from build123d import *

# Parameters (mm, degrees)
F0_W     = 9
F0_H     = 5.1
F1_DEPTH = 0.5
F2_SIZE  = 0.5
F3_SIZE  = 0.1


with BuildPart() as f1:
    # F0 (on Front) → F1 (new body, symmetric)
    with BuildSketch(Plane.XZ):
        with Locations((4.5, 2.55)):
            Rectangle(F0_W, F0_H)
    extrude(amount=F1_DEPTH, both=True)

    # F2
    f2_edges = [f1.edges().sort_by_distance(p)[0] for p in [
        (4.5, 0.5, 0),
    ]]
    chamfer(f2_edges, length=F2_SIZE)

    # F3
    f3_edges = [f1.edges().sort_by_distance(p)[0] for p in [
        (4.5, -0.5, 0),
    ]]
    chamfer(f3_edges, length=F3_SIZE)


solid = f1.part
Design review of the part built by this model. Coordinates are the model's own, in mm. Give positions to 0.01 mm unless a question says otherwise; leave off trailing zeros. Loops run counter-clockwise (first coordinate to the right, second up) from the corner with the lowest first, then second, coordinate; pieces in that order, holes last. Notation, with made-up numbers: M 69,64.25 L 91,64.25 A17 ccw 91,71.25 Z; hole C -23.5,7 d5. An arc over 180 degrees is marked long. One line per question, with ' | ' between items. Start each with the question number.
1. To check wall thickness, follow L1, parallel to Y at x = 8.75, z = 0.4; L2, parallel to Z at x = 1.5, y = 0.05; L3, parallel to Z at x = 6.5, y = 0.35. State the ranges of each line that lie inside material, in increasing order.
2. The part is to be moulded in two halves that separate along Z. For faces 1 (the face through (4, 0, 5.1)), 2 (the face through (4, -0.5, 3)), say which applies: released by +Z, released by -Z, zero draft, split by the parting line, or undercut.
3. Add section B-B (y = 0.4). Write out the cut boundary in (x, z).
4. Add section A-A (x = 4). Write out the cut boundary in (y, z), plus the area to 3 significant figures.
Worked out:
1) L1: y = -0.5 to 0.4 | L2: z = 0.05 to 5.1 | L3: z = 0.35 to 5.1
2) face 1: released by +Z | face 2: zero draft
3) outline: M 0,0.4 L 9,0.4 L 9,5.1 L 0,5.1 Z
4) outline: M -0.5,0.1 L -0.4,0 L 0,0 L 0.5,0.5 L 0.5,5.1 L -0.5,5.1 Z | area: 4.97 mm²
